The model under review builds one solid part; all positions refer to its coordinate system, in mm. Face numbers are marked on the shaded views. Round coordinates to 2 decimals unless told otherwise and drop trailing zeros. Order: outer loops, then holes, each group sorted by start corner. A loop starts at its lowest first (then second) coordinate and runs counter-clockwise, first axis right, second up.
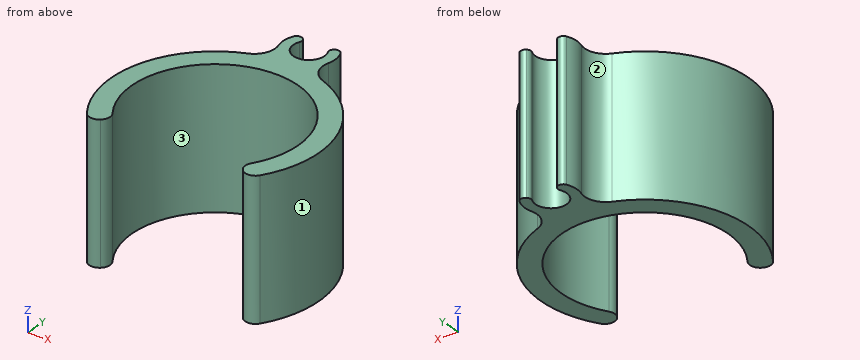
```python
from build123d import *

# Parameters (mm, degrees)
F1_DEPTH = 20


with BuildPart() as f1:
    # F0 (on Top) → F1 (new body)
    with BuildSketch(Plane.XY):
        with BuildLine():
            ThreePointArc((-9.992663, -6.644297), (0, 12), (9.992663, -6.644297))
            ThreePointArc((9.992663, -6.644297), (9.757043, -7.68851), (10.277565, -8.623901))
            ThreePointArc((10.277565, -8.623901), (11.455422, -8.959537), (12.490829, -8.305371))
            ThreePointArc((12.490829, -8.305371), (14.292312, 4.553001), (5.385165, 14))
            ThreePointArc((5.385165, 14), (3.767759, 15.480909), (3.59011, 17.666667))
            ThreePointArc((3.59011, 17.666667), (3.73912, 19.035446), (3.384061, 20.365745))
            ThreePointArc((3.384061, 20.365745), (2.866238, 20.77555), (2.225158, 20.617129))
            ThreePointArc((2.225158, 20.617129), (1.974294, 20.201585), (2.030437, 19.719447))
            ThreePointArc((2.030437, 19.719447), (0, 16.5), (-2.030437, 19.719447))
            ThreePointArc((-2.030437, 19.719447), (-1.974294, 20.201585), (-2.225158, 20.617129))
            ThreePointArc((-2.225158, 20.617129), (-2.866238, 20.77555), (-3.384061, 20.365745))
            ThreePointArc((-3.384061, 20.365745), (-3.73912, 19.035446), (-3.59011, 17.666667))
            ThreePointArc((-3.59011, 17.666667), (-3.767759, 15.480909), (-5.385165, 14))
            ThreePointArc((-5.385165, 14), (-14.292312, 4.553001), (-12.490829, -8.305371))
            ThreePointArc((-12.490829, -8.305371), (-11.455422, -8.959537), (-10.277565, -8.623901))
            ThreePointArc((-10.277565, -8.623901), (-9.757043, -7.68851), (-9.992663, -6.644297))
        make_face()
    extrude(amount=F1_DEPTH)


solid = f1.part
```
(1) Consider section C-C (z = 15.25). Write out the cut boundary in (x, y).
Data:
outline: (-12.49, -8.31) arc R1.5 ccw to (-9.99, -6.64) arc R12 cw (long way) to (9.99, -6.64) arc R1.5 ccw to (12.49, -8.31) arc R15 ccw to (5.39, 14) arc R3 cw to (3.59, 17.67) arc R3.75 ccw to (3.38, 20.37) arc R0.75 ccw to (2.23, 20.62) arc R0.75 ccw to (2.03, 19.72) arc R2.25 cw (long way) to (-2.03, 19.72) arc R0.75 ccw to (-2.23, 20.62) arc R0.75 ccw to (-3.38, 20.37) arc R3.75 ccw to (-3.59, 17.67) arc R3 cw to (-5.39, 14) arc R15 ccw to start
(2) Insertion check: pin 1 (4 mm diameter, centred on x = -7.5, y = 12, fed in from -Z); pin 2 (6 mm diameter, centred on y = 12, z = 11.5, fed in from -X); pin 3 (3 mm diameter, centred on x = -9, z = 13.5, fed in from -Y); pin 4 (4 mm diameter, centred on y = 7, z = 12, fed in from +X). Each pin has a flat end and moves straight along its axis. Give the tip position at first contact, or say it passes through.
Data:
pin 1: stops at z = 0
pin 2: stops at x = -12
pin 3: stops at y = -8.78
pin 4: stops at x = 14.14
(3) Consider section A-A (y = 0). Write out the cut boundary in (x, z), and give its area (3 significant figures).
Data:
outline: (-15, 0) - (-12, 0) - (-12, 20) - (-15, 20) - close; (12, 0) - (15, 0) - (15, 20) - (12, 20) - close
area: 120 mm2
(4) To check wall thickness, follow probe 1 along X at (y, z) = (0, 11.5); probe 2 along X at (y, z) = (18.75, 6.5); probe 3 along Y at (x, z) = (0, 9.25). State the ranges of each line that lie inside material, in increasing order.
Data:
probe 1: x = -15 to -12, 12 to 15
probe 2: x = -3.75 to -2.25, 2.25 to 3.75
probe 3: y = 12 to 16.5
(5) Draft analysis for pull direction X (two halves, no side actions). For the marked faces 1, 2 and 3, state which applies: pulls with the +X half, pulls with the -X half, needs draft (parallel to the pull), parting line crosses it, or undercut.
Data:
face 1: pulls with the +X half
face 2: pulls with the -X half
face 3: undercut
(6) Consider section B-B (x = 11). Write out the cut boundary in (y, z), and give its area (3 significant figures).
Data:
outline: (-8.96, 0) - (-4.8, 0) - (-4.8, 20) - (-8.96, 20) - close; (4.8, 0) - (10.2, 0) - (10.2, 20) - (4.8, 20) - close
area: 191 mm2
(7) Consider section D-D (x = 0). Write out the cut boundary in (y, z), and give its area (3 significant figures).
Data:
outline: (12, 0) - (16.5, 0) - (16.5, 20) - (12, 20) - close
area: 90.0 mm2
